Part print with two shaded views. Sizes in mm from the minimum x, y, z corner. A direction names the side the tool comes from. Coordinates: 2 decimals unless noted, no trailing zeros. Loops run counter-clockwise (first coordinate to the right, second up) from the corner with the lowest first, then second, coordinate; pieces in that order, holes last.
(1) Slice it at B-B (x = 15). Give the cut face in (y, z).
(2) Slice it at D-D (z = 20.5). Give the cut face in (x, y).
(3) Slice it at C-C (y = 103.5). Give the cut face in (x, z).
(4) Tool access for the marked faces 1 and 2: list every direction of +Z, -Z, +X, -X, +Y, -Y with a clear straight run to the whole face (end or side of a thin tool).
(5) Wall check: L1, parallel to Y at x = 15, z = 27.05; L2, parallel to Z at x = 2.65, y = 80; L3, parallel to Z at x = 10, y = 19.5. Give the ranges that are in metal, low to high.
(6) Slice it at A-A (y = 185). Give the cut face in (x, z), and give its area (3 significant figures).
(7) Flat gauge pins, fed straight in: P1, Ø1, axis at x = 11, y = 160, coming from the -Z side; P2, Ø5, axis at y = 180, z = 15, coming from the +X side. Where does each tip first touch, or does it go through?
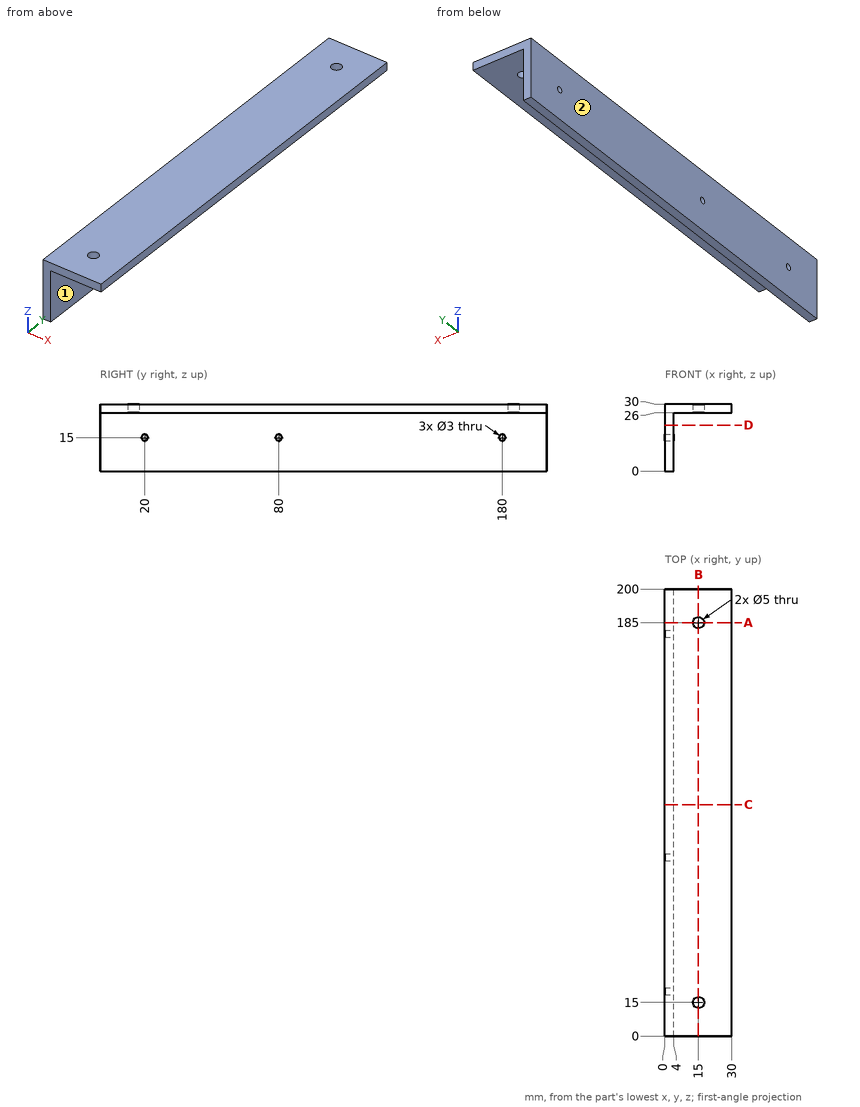
Response values:
1. outline: (0, 26) - (12.5, 26) - (12.5, 30) - (0, 30) - close; (17.5, 26) - (182.5, 26) - (182.5, 30) - (17.5, 30) - close; (187.5, 26) - (200, 26) - (200, 30) - (187.5, 30) - close
2. outline: (0, 0) - (4, 0) - (4, 200) - (0, 200) - close
3. outline: (0, 0) - (4, 0) - (4, 26) - (30, 26) - (30, 30) - (0, 30) - close
4. face 1: -Z, +X, +Y, -Y
4. face 2: +Z, -Z, -X, +Y, -Y
5. L1: y = 0 to 12.5, 17.5 to 182.5, 187.5 to 200
5. L2: z = 0 to 13.5, 16.5 to 30
5. L3: z = 26 to 30
6. outline: (0, 0) - (4, 0) - (4, 26) - (12.5, 26) - (12.5, 30) - (0, 30) - close; (17.5, 26) - (30, 26) - (30, 30) - (17.5, 30) - close
6. area: 204 mm2
7. P1: stops at z = 26
7. P2: stops at x = 4
